```python
from build123d import *

# Parameters (mm, degrees)
F0_W        = 78.74
F0_H        = 76.2
F1_DEPTH    = 33.02
F2_T        = -2.54
F3_T4_DEPTH = 73.66
F4_SIZE     = 25.4


# Not quite as in the source:
# - a fillet or chamfer that OpenCascade refuses, or shapes differently, is made with other operations: its cross-section is extruded or revolved along the edge and cut away or added


with BuildPart() as f1:
    # F0 (on Right) → F1 (new body)
    with BuildSketch(Plane.YZ):
        with Locations((-1.4558544075, -12.2276971856)):
            Rectangle(F0_W, F0_H)
    extrude(amount=F1_DEPTH)

    # F2
    f2_openings = [f1.faces().sort_by_distance(p)[0] for p in [
        (33.02, -1.455854, -12.227697),
        (16.51, -1.455854, 25.872303),
    ]]
    offset(amount=F2_T, openings=f2_openings)

    # F3: chamfer of 30.48 on 1 edges, made by hand


with BuildPart() as f3_tool2:
    # F3_s3 → F3_t4 (new body)
    with BuildSketch(Plane.XZ.offset(38.2858544075)):
        with BuildLine():
            Line((33.8821045876, -79.1298017732), (1.6778954124, -46.925592598))
            Line((1.6778954124, -46.925592598), (1.6778954124, -46.315992598))
            ThreePointArc((1.6778954124, -46.315992598), (17.3489477062, -47.1780971856), (33.02, -47.1780971856))
            Line((33.02, -47.1780971856), (33.6296, -47.7876971856))
            ThreePointArc((33.6296, -47.7876971856), (33.6296, -63.4587494794), (34.4917045876, -79.1298017732))
            Line((34.4917045876, -79.1298017732), (33.8821045876, -79.1298017732))
        make_face()
    extrude(amount=-F3_T4_DEPTH)

    split(bisect_by=Plane.YZ.offset(2.54), keep=Keep.TOP)


with BuildPart() as f1_1:
    add(f1.part)

    # F3_t1: cut F3_tool2
    add(f3_tool2.part, mode=Mode.SUBTRACT)

    # F4
    f4_edges = [f1_1.edges().sort_by_distance(p)[0] for p in [
        (33.02, -39.555854, -50.327697),
        (33.02, 36.644146, -50.327697),
    ]]
    chamfer(f4_edges, length=F4_SIZE)


solid = f1_1.part
```
Input: part model. Units: mm. Frame: model coordinates. A direction names the side the tool comes from. Coordinates: 2 decimals unless noted, no trailing zeros. Write each loop counter-clockwise with the first axis right and the second up, starting at its lowest first coordinate (ties: lowest second). Pieces come first, ordered by that corner, then holes. Notation, with made-up numbers: (26, 53) - (68, 53) arc R29 cw to (68, 80) - close; hole circle Ø8 at (87, -35). An arc over 180 degrees is marked (long way). Put each result on its own line as item: value. Start each with the question number.
1) Contact query for flat-ended pins moving along their axis: pin 1 (12 mm diameter, centred on x = 11.5, y = 21, fed in from +Z); pin 2 (12 mm diameter, centred on x = 10.5, y = 18.5, fed in from +Z); pin 3 (10 mm diameter, centred on y = -33, z = 2.5, fed in from +X). Output: stop coordinate, or through.
2) Cut plane A-A (z = 12.5). Return the cut outline in (x, y), plus the area to 3 significant figures.
3) Cut plane B-B (x = 15). Return the cut outline in (y, z), plus the area to 3 significant figures.
4) Mould query, pull axis Y, two halves, no side actions, for faces 3 (the face through (18, -38.286, -3)), 4 (the face through (20.14, -39.57, -37.81)), 5 (the face through (16, -40.826, -4)). Classes: pulls with the +Y half, pulls with the -Y half, needs draft (parallel to the pull), parting line crosses it, or undercut.
5) Cut plane C-C (y = -21.5). Return the cut outline in (x, z).
6) Reachability of faces 1 (the face through (2, -2, -50.328)), 2 (the face through (3.83, -1.97, -49.08)) from +Z, -Z, +X, -X, +Y, -Y: full face, straight path, thin tool, end or side. Return the list, or none.
7) Cut plane D-D (x = 30.5). Return the cut outline in (y, z), plus the area to 3 significant figures.
8) Ray query, L1, parallel to Y at x = 25.5, z = -8.5; L2, parallel to X at y = -13, z = 22.5; L3, parallel to Z at x = 3.5, y = 5.5. Return the intervals inside material, ascending.
Resolved:
1. pin 1: passes through
1. pin 2: stops at z = -49.75
1. pin 3: stops at x = 2.54
2. outline: (0, -40.83) - (33.02, -40.83) - (33.02, -38.29) - (2.54, -38.29) - (2.54, 35.37) - (33.02, 35.37) - (33.02, 37.91) - (0, 37.91) - close
2. area: 355 mm2
3. outline: (-40.83, -42.95) - (-38.29, -42.95) - (-38.29, 25.87) - (-40.83, 25.87) - close; (35.37, -42.95) - (37.91, -42.95) - (37.91, 25.87) - (35.37, 25.87) - close
3. area: 350 mm2
4. face 3: undercut
4. face 4: needs draft
4. face 5: pulls with the -Y half
5. outline: (0, -50.33) - (5.08, -50.33) - (2.54, -47.79) - (2.54, 25.87) - (0, 25.87) - close
6. face 1: -Z, +X, -X, +Y, -Y
6. face 2: +Z, +X
7. outline: (-40.83, -27.45) - (-38.29, -27.45) - (-38.29, 25.87) - (-40.83, 25.87) - close; (35.37, -27.45) - (37.91, -27.45) - (37.91, 25.87) - (35.37, 25.87) - close
7. area: 271 mm2
8. L1: y = -40.83 to -38.29, 35.37 to 37.91
8. L2: x = 0 to 2.54
8. L3: z = -50.33 to -48.75
